Could you check a few things on this model? Use its own coordinates, in mm. Face numbers are marked on the shaded views. A direction names the side the tool comes from. Give positions to 0.01 mm unless a question says otherwise; leave off trailing zeros. Write each loop counter-clockwise with the first axis right and the second up, starting at its lowest first coordinate (ties: lowest second). Pieces come first, ordered by that corner, then holes. Notation, with made-up numbers: (7, 44) - (47, 44) arc R21 cw to (47, 71) - close; hole circle Ø5 at (-15.5, -8). An arc over 180 degrees is marked (long way). Answer in a Markdown table with one row per item.
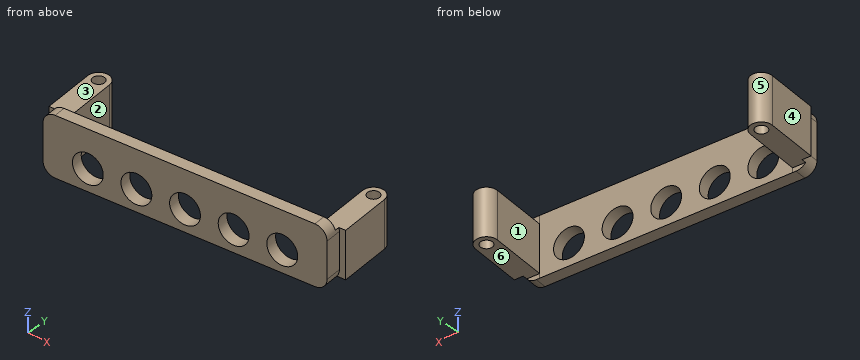
from build123d import *

# Parameters (mm, degrees)
F1_DEPTH = 12.8
F3_DEPTH = 3.5
F4_W     = 18.9070843756
F4_H     = 1.75
F4_W_2   = 22.2780885547
F4_H_2   = 0.95
F5_DEPTH = 62.4295319173
F7_D     = 2.5
F9_D     = 6.35


with BuildPart() as f1:
    # F0 (on Top) → F1 (new body)
    with BuildSketch(Plane.XY):
        with BuildLine():
            ThreePointArc((-27.292256768, 11.945013416), (-29.7470947197, 13.9695554954), (-31.771636799, 11.5147175437))
            Line((-31.771636799, 11.5147175437), (-30.385127877, -2.918840334))
            Line((-30.385127877, -2.918840334), (30.385127877, 2.918840334))
            Line((30.385127877, 2.918840334), (28.9986189551, 17.3523982117))
            ThreePointArc((28.9986189551, 17.3523982117), (26.5437810034, 19.3769402911), (24.5192389241, 16.9221023394))
            Line((24.5192389241, 16.9221023394), (25.6666945836, 4.9770889233))
            Line((25.6666945836, 4.9770889233), (-26.1448011084, 0))
            Line((-26.1448011084, 0), (-27.292256768, 11.945013416))
        make_face()
    extrude(amount=F1_DEPTH)

    # F2 (on face) → F3 (cut)
    with BuildSketch(Plane(origin=(0, 0, 0), x_dir=(0.9954177847, 0.095621305, 0), z_dir=(0.095621305, -0.9954177847, 0))):
        with BuildLine():
            ThreePointArc((-29.225, 10.3), (-28.492766953, 12.067766953), (-26.725, 12.8))
            Line((-26.725, 12.8), (-30.525, 12.8))
            Line((-30.525, 12.8), (-30.525, 0))
            Line((-30.525, 0), (-26.725, 0))
            ThreePointArc((-26.725, 0), (-28.492766953, 0.732233047), (-29.225, 2.5))
            Line((-29.225, 2.5), (-29.225, 10.3))
        make_face()
        with BuildLine():
            Line((30.525, 12.8), (26.725, 12.8))
            ThreePointArc((26.725, 12.8), (28.492766953, 12.067766953), (29.225, 10.3))
            Line((29.225, 10.3), (29.225, 2.5))
            ThreePointArc((29.225, 2.5), (28.492766953, 0.732233047), (26.725, 0))
            Line((26.725, 0), (30.525, 0))
            Line((30.525, 0), (30.525, 12.8))
        make_face()
    extrude(amount=-F3_DEPTH, mode=Mode.SUBTRACT)

    # F4 (on face) → F5 (cut, through all)
    with BuildSketch(Plane(origin=(30.385127877, 2.918840334, 0), x_dir=(-0.095621305, 0.9954177847, 0), z_dir=(0.9954177847, 0.095621305, 0))):
        with Locations((11.9535421878, 11.925)):
            Rectangle(F4_W, F4_H)
        with Locations((13.6390442774, 0.475)):
            Rectangle(F4_W_2, F4_H_2)
    extrude(amount=-F5_DEPTH, mode=Mode.SUBTRACT)

    # F7 (through all)
    with Locations(Plane(origin=(0, 0, 0.95), x_dir=(1, 0, 0), z_dir=(0, 0, -1))):
        with Locations((26.7589289396, -17.1372502756), (-29.5319467835, -11.7298654799)):
            Hole(F7_D / 2)

    # F9 (through all)
    with Locations(Plane(origin=(0, 0, 0), x_dir=(0.9954177847, 0.095621305, 0), z_dir=(0.095621305, -0.9954177847, 0))):
        with Locations((-20, 4.69), (-10, 4.69), (0, 4.69), (10, 4.69), (20, 4.69)):
            Hole(F9_D / 2)


solid = f1.part
1) Imagine slicing it at D-D (x = -14). List the corners of the cut face in (y, z) for me, then the cut area to 3 significant figures.
Check values:
| item | result |
|---|---|
| outline | (-1.34, 0) - (1.17, 0) - (1.17, 12.8) - (-1.34, 12.8) - close |
| area | 32.1 mm2 |
2) If I drill on line 1 (X direction, y = 0.75, z = 6.5); line 2 (Z direction, x = -11.5, y = 0.75); line 3 (Y direction, x = 27, z = 2), over which ranges is the centre line in solid material (lowest first)?
Check values:
| item | result |
|---|---|
| line 1 | x = -30.74 to -26.22, -17.54 to -12.74, -7.5 to -2.69, 2.55 to 7.35 |
| line 2 | z = 0 to 1.83, 7.55 to 12.8 |
| line 3 | y = 2.59 to 15.91, 18.36 to 19.37 |
3) Imagine slicing it at B-B (y = 8.75). List the corners of the cut face in (x, z) for me, then the cut area to 3 significant figures.
Check values:
| item | result |
|---|---|
| outline | (-31.51, 0.95) - (-26.99, 0.95) - (-26.99, 11.05) - (-31.51, 11.05) - close; (25.3, 0.95) - (29.82, 0.95) - (29.82, 11.05) - (25.3, 11.05) - close |
| area | 91.3 mm2 |
4) Imagine slicing it at A-A (z = 6.5). State how many separate pieces and enclosed holes the cut face has, then the cut area to 3 significant figures.
Check values:
| item | result |
|---|---|
| separate pieces | 6 |
| enclosed holes | 2 |
| area | 192 mm2 |
5) Will these pins go through, and if not, where does the flat tip stop? P1, Ø8, axis at x = 16, y = 5.5, coming from the +Z side; P2, Ø6, axis at x = 27.5, y = 15, coming from the +Z side; P3, Ø4, axis at x = 26.76, y = 17.14, coming from the -Z side; P4, Ø3, axis at y = 7.5, z = 8, coming from the -X side.
Check values:
| item | result |
|---|---|
| P1 | stops at z = 12.8 |
| P2 | stops at z = 11.05 |
| P3 | stops at z = 0.95 |
| P4 | stops at x = -31.53 |
6) On a 3-axis mill with a long thin cutter (end or side, diameter ignored), from which of +Z, -Z, +X, -X, +Y, -Y can I reach the whole of each face in a straight line? I mean the marked faces 1, 2 and 3. Say none if no direction works.
Check values:
| item | result |
|---|---|
| face 1 | +Z, -Z |
| face 2 | +Z, -Z, +Y |
| face 3 | +Z, -X, +Y |
7) We'd pull the mould along X, two halves only. Please class the marked faces 4, 5 and 6: +X half, -X half, draft (parallel to the pull), parting line (faces both ways), or undercut.
Check values:
| item | result |
|---|---|
| face 4 | -X half |
| face 5 | undercut |
| face 6 | draft |
